For this review, take the finished solid that the model builds, in its own axes (mm). Face numbers are marked on the shaded views. A direction names the side the tool comes from. Give positions to 0.01 mm unless a question says otherwise; leave off trailing zeros. Write each loop counter-clockwise with the first axis right and the second up, starting at its lowest first coordinate (ties: lowest second). Pieces come first, ordered by that corner, then holes.
1) Wall thickness on line 1 along Y through (x, z) = (-15, 0.6); line 2 along Z through (x, y) = (-11.5, 5.5); line 3 along X through (y, z) = (-4.75, 13.75): over which ranges is each line inside the solid? List them lowest first.
2) We need section A-A on y = 0. Give the boundary of the cut face in (x, z), and give its area (3 significant figures).
3) We need section C-C on x = 0. Give the boundary of the cut face in (y, z).
4) Machinability: for the marked faces 1 and 2, which of the approach directions +Z, -Z, +X, -X, +Y, -Y give a long, thin tool a straight path to every point of the face, cutting with its end or side? Answer none if there is none.
5) For P1, Ø8, axis at x = 9, z = 13.5, coming from the -Y side; P2, Ø10, axis at x = 15, y = -3, coming from the +Z side; P3, Ø6, axis at x = -3.5, z = 8.5, coming from the +Y side; P4, Ø2.5, axis at x = 15, y = 0, coming from the -Z side, all flat-tipped, find the tip position at first contact; note any pin that passes through.
6) We need section B-B on x = -15. Give the boundary of the cut face in (y, z), and give its area (3 significant figures).
7) We need section D-D on y = 5.5. Give the boundary of the cut face in (x, z).
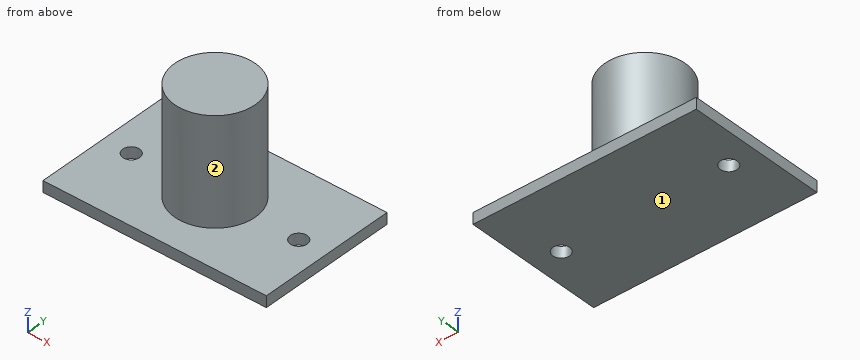
from build123d import *

# Parameters (mm, degrees)
SKETCH1_W           = 40
SKETCH1_H           = 25
SKETCH1_R           = 1.5
BOSS_EXTRUDE1_DEPTH = 2
SKETCH2_R           = 7.2
BOSS_EXTRUDE2_DEPTH = 19


with BuildPart() as part:
    # Sketch1 → Boss-Extrude1 (new body)
    with BuildSketch(Plane.XY):
        Rectangle(SKETCH1_W, SKETCH1_H)
        with Locations((15, 0)):
            Circle(SKETCH1_R, mode=Mode.SUBTRACT)
        with Locations((-15, 0)):
            Circle(SKETCH1_R, mode=Mode.SUBTRACT)
    extrude(amount=BOSS_EXTRUDE1_DEPTH)

    # Sketch2 → Boss-Extrude2 (add)
    with BuildSketch(Plane.XY.offset(2)):
        Circle(SKETCH2_R)
    extrude(amount=BOSS_EXTRUDE2_DEPTH)


solid = part.part
Results list:
1. line 1: y = -12.5 to -1.5, 1.5 to 12.5
1. line 2: z = 0 to 2
1. line 3: x = -5.41 to 5.41
2. outline: (-20, 0) - (-16.5, 0) - (-16.5, 2) - (-20, 2) - close; (-13.5, 0) - (13.5, 0) - (13.5, 2) - (7.2, 2) - (7.2, 21) - (-7.2, 21) - (-7.2, 2) - (-13.5, 2) - close; (16.5, 0) - (20, 0) - (20, 2) - (16.5, 2) - close
2. area: 342 mm2
3. outline: (-12.5, 0) - (12.5, 0) - (12.5, 2) - (7.2, 2) - (7.2, 21) - (-7.2, 21) - (-7.2, 2) - (-12.5, 2) - close
4. face 1: -Z, +X, -X, +Y, -Y
4. face 2: +Z
5. P1: stops at y = -5.18
5. P2: stops at z = 2
5. P3: stops at y = 7.18
5. P4: passes through
6. outline: (-12.5, 0) - (-1.5, 0) - (-1.5, 2) - (-12.5, 2) - close; (1.5, 0) - (12.5, 0) - (12.5, 2) - (1.5, 2) - close
6. area: 44.0 mm2
7. outline: (-20, 0) - (20, 0) - (20, 2) - (4.65, 2) - (4.65, 21) - (-4.65, 21) - (-4.65, 2) - (-20, 2) - close
